Design review of the part built by this model. Coordinates are the model's own, in mm. Face numbers are marked on the shaded views. Coordinates: 2 decimals unless noted, no trailing zeros. Loops run counter-clockwise (first coordinate to the right, second up) from the corner with the lowest first, then second, coordinate; pieces in that order, holes last. Notation, with made-up numbers: (-27.75, 4) - (19.25, 4) arc R29 cw to (19.25, 31) - close; hole circle Ø7 at (-1, 69.25). An arc over 180 degrees is marked (long way). Answer in a Markdown table with one row per item. Add a question column.
(1) We need section A-A, the plane z = 0. Write out the cut boundary in (x, y), plus the area to 3 significant figures.
(2) We need section C-C, the plane z = -38. Write out the cut boundary in (x, y).
(3) Clearance check with a flat-ended pin moving along its axis: pin 1 (5 mm diameter, centred on x = -34.5, z = 11, fed in from +Y). State where the tip first meets the part, or that it passes through.
(4) We need section B-B, the plane x = -4. Write out the cut boundary in (y, z), plus the area to 3 significant figures.
(5) The part is to be moulded in two halves that separate along X. For the marked faces 1, 2, 3 and 4, say which applies: released by +X, released by -X, zero draft, split by the parting line, or undercut.
(6) To check wall thickness, follow L1, parallel to X at y = 6.35, z = 0; L2, parallel to Y at x = -51, z = 37; L3, parallel to Y at x = -7, z = -7. State the ranges of each line that lie inside material, in increasing order. Write a range as [from, to].
(7) We need section D-D, the plane x = -24.5. Write out the cut boundary in (y, z).
from build123d import *

# Parameters (mm, degrees)
EXTRUDE_1_DEPTH     = 10
CUT_EXTRUDE_START   = -3
CUT_EXTRUDE_1_DEPTH = 3
SKETCH_3_R          = 20
CUT_EXTRUDE_2_DEPTH = 6
CUT_EXTRUDE_3_DEPTH = 1


with BuildPart() as part:
    # 草图1 → 凸台-拉伸1 (new body)
    with BuildSketch(Plane(origin=(0, 0, 0), x_dir=(1, 0, 0), z_dir=(0, 1, 0))):
        with BuildLine():
            Line((-61.551724138, 50), (18.448275862, 50))
            ThreePointArc((18.448275862, 50), (25.519343674, 47.071067812), (28.448275862, 40))
            Line((28.448275862, 40), (28.448275862, -40))
            ThreePointArc((28.448275862, -40), (25.519343674, -47.071067812), (18.448275862, -50))
            Line((18.448275862, -50), (-61.551724138, -50))
            ThreePointArc((-61.551724138, -50), (-68.62279195, -47.071067812), (-71.551724138, -40))
            Line((-71.551724138, -40), (-71.551724138, 40))
            ThreePointArc((-71.551724138, 40), (-68.62279195, 47.071067812), (-61.551724138, 50))
        make_face()
    extrude(amount=EXTRUDE_1_DEPTH)

    # 草图2 → 切除-拉伸1 (cut)
    with BuildSketch(Plane(origin=(0, 10, 0), x_dir=(1, 0, 0), z_dir=(0, 1, 0)).offset(CUT_EXTRUDE_START)):
        with BuildLine():
            Line((-21.551724138, 10), (-61.551724138, 50))
            ThreePointArc((-61.551724138, 50), (-63.154135948, 49.870778915), (-64.715134679, 49.486455279))
            Line((-64.715134679, 49.486455279), (-21.551724138, 6.323044738))
            Line((-21.551724138, 6.323044738), (21.611686403, 49.486455279))
            ThreePointArc((21.611686403, 49.486455279), (20.050687672, 49.870778915), (18.448275862, 50))
            Line((18.448275862, 50), (-21.551724138, 10))
        make_face()
        with BuildLine():
            Line((-21.551724138, -10), (18.448275862, -50))
            ThreePointArc((18.448275862, -50), (20.050687672, -49.870778915), (21.611686403, -49.486455279))
            Line((21.611686403, -49.486455279), (-21.551724138, -6.323044738))
            Line((-21.551724138, -6.323044738), (-64.715134679, -49.486455279))
            ThreePointArc((-64.715134679, -49.486455279), (-63.154135948, -49.870778915), (-61.551724138, -50))
            Line((-61.551724138, -50), (-21.551724138, -10))
        make_face()
    extrude(amount=CUT_EXTRUDE_1_DEPTH, mode=Mode.SUBTRACT)

    # 草图3 → 切除-拉伸2 (cut)
    with BuildSketch(Plane(origin=(0, 10, 0), x_dir=(1, 0, 0), z_dir=(0, 1, 0))):
        with Locations(Location((-21.551724138, 0, 0), (0, 0, 270))):
            Circle(SKETCH_3_R)
    extrude(amount=-CUT_EXTRUDE_2_DEPTH, mode=Mode.SUBTRACT)

    # 草图5 → 切除-拉伸3 (cut)
    with BuildSketch(Plane(origin=(0, 10, 0), x_dir=(1, 0, 0), z_dir=(0, 1, 0))):
        Polygon((-21.551724138, 43.940949844), (-29.190091611, 36.302582371), (-13.913356665, 36.302582371), align=None)
    extrude(amount=-CUT_EXTRUDE_3_DEPTH, mode=Mode.SUBTRACT)


solid = part.part
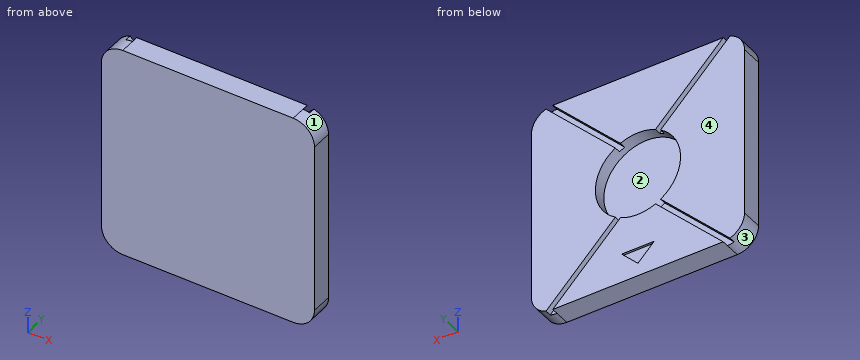
Responses:
| question | item | result |
|---|---|---|
| 1 | outline | (-71.55, 0) - (28.45, 0) - (28.45, 10) - (-1.55, 10) - (-1.55, 4) - (-41.55, 4) - (-41.55, 10) - (-71.55, 10) - close |
| 1 | area | 760 mm2 |
| 2 | outline | (-71.55, 0) - (28.45, 0) - (28.45, 10) - (10.13, 10) - (10.13, 7) - (6.45, 7) - (6.45, 10) - (-15.61, 10) - (-15.61, 9) - (-27.49, 9) - (-27.49, 10) - (-49.55, 10) - (-49.55, 7) - (-53.23, 7) - (-53.23, 10) - (-71.55, 10) - close |
| 3 | pin 1 | stops at y = 4 |
| 4 | outline | (0, -50) - (10, -50) - (10, -27.55) - (7, -27.55) - (7, -23.87) - (10, -23.87) - (10, -9.59) - (4, -9.59) - (4, 9.59) - (10, 9.59) - (10, 23.87) - (7, 23.87) - (7, 27.55) - (10, 27.55) - (10, 50) - (0, 50) - close |
| 4 | area | 863 mm2 |
| 5 | face 1 | released by +X |
| 5 | face 2 | undercut |
| 5 | face 3 | released by -X |
| 5 | face 4 | zero draft |
| 6 | L1 | x = [-71.55, -41.55], [-1.55, 28.45] |
| 6 | L2 | y = [0, 7] |
| 6 | L3 | y = [0, 4] |
| 7 | outline | (0, -50) - (10, -50) - (10, -40.99) - (9, -40.99) - (9, -36.3) - (10, -36.3) - (10, -19.78) - (4, -19.78) - (4, 19.78) - (10, 19.78) - (10, 50) - (0, 50) - close |
